The model under review builds one solid part; all positions refer to its coordinate system, in mm. Face numbers are marked on the shaded views. A direction names the side the tool comes from. Coordinates: 2 decimals unless noted, no trailing zeros. Loops run counter-clockwise (first coordinate to the right, second up) from the corner with the lowest first, then second, coordinate; pieces in that order, holes last. Notation, with made-up numbers: M 83.5,9 L 107.5,9 A26 cw 107.5,47 Z; hole C 80,20.5 d6. An arc over 180 degrees is marked long. Return JSON: item names as keys, results as strings.
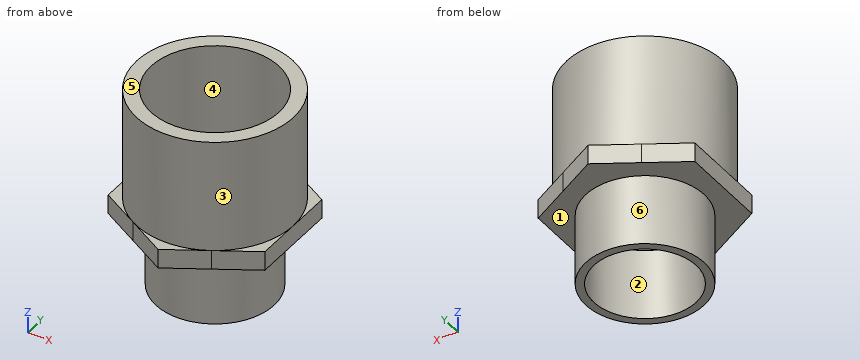
```python
from build123d import *

# Parameters (mm, degrees)
F3_DEPTH = 6


with BuildPart() as f1:
    # F0 (on Front) → F1 (revolve)
    with BuildSketch(Plane.XZ):
        Polygon((-18.5, 0), (-16, 0), (-16, 22), (-20, 28), (-20, 63), (-24.5, 63), (-24.5, 28), (-24.5, 22), (-18.5, 22), align=None)
    revolve(axis=Axis((0, 0, 64.797089), (0, 0, 1)))

    # F2 (on face) → F3 (join)
    with BuildSketch(Plane(origin=(0, 0, 22), x_dir=(1, 0, 0), z_dir=(0, 0, -1))):
        with BuildLine():
            Line((24.5, -14.145082), (24.5, 0))
            ThreePointArc((24.5, 0), (21.217622, -12.25), (12.25, -21.217622))
            Line((12.25, -21.217622), (24.5, -14.145082))
        make_face()
        with BuildLine():
            ThreePointArc((12.25, 21.217622), (21.217622, 12.25), (24.5, 0))
            Line((24.5, 0), (24.5, 14.145082))
            Line((24.5, 14.145082), (12.25, 21.217622))
        make_face()
        with BuildLine():
            ThreePointArc((-12.249999, 21.217623), (0, 24.5), (12.25, 21.217622))
            Line((12.25, 21.217622), (0, 28.290163))
            Line((0, 28.290163), (-12.249999, 21.217623))
        make_face()
        with BuildLine():
            Line((0, -28.290163), (12.25, -21.217622))
            ThreePointArc((12.25, -21.217622), (0, -24.5), (-12.25, -21.217622))
            Line((-12.25, -21.217622), (0, -28.290163))
        make_face()
        with BuildLine():
            ThreePointArc((-24.5, 0), (-21.217622, 12.25), (-12.249999, 21.217623))
            Line((-12.249999, 21.217623), (-24.5, 14.145082))
            Line((-24.5, 14.145082), (-24.5, 0))
        make_face()
        with BuildLine():
            Line((-24.5, -14.145082), (-12.25, -21.217622))
            ThreePointArc((-12.25, -21.217622), (-21.217622, -12.25), (-24.5, 0))
            Line((-24.5, 0), (-24.5, -14.145082))
        make_face()
    extrude(amount=-F3_DEPTH)

    # F4 (on Front) → F5 (revolve, cut)
    with BuildSketch(Plane.XZ):
        Polygon((-20, 28), (-16, 22), (0, 22), (0, 28), (-12.25, 28), align=None)
    revolve(axis=Axis((0, 0, 34.552477), (0, 0, 1)), mode=Mode.SUBTRACT)


solid = f1.part
```
1. Add section B-B on y = -23.5. Give the boundary of the cut face in (x, z).
Check values:
{"outline": "M -8.3,22 L 8.3,22 L 8.3,28 L 6.93,28 L 6.93,63 L -6.93,63 L -6.93,28 L -8.3,28 Z"}
2. The part is to be moulded in two halves that separate along X. For the marked faces 4, 5 and 6, say which applies: released by +X, released by -X, zero draft, split by the parting line, or undercut.
Check values:
{"face 4": "undercut", "face 5": "zero draft", "face 6": "split by the parting line"}
3. Add section D-D on z = 4. Give the boundary of the cut face in (x, y).
Check values:
{"outline": "C 0,0 d37; hole C 0,0 d32"}
4. Add section C-C on z = 51.5. Give the boundary of the cut face in (x, y).
Check values:
{"outline": "C 0,0 d49; hole C 0,0 d40"}
5. To check wall thickness, follow line 1 (X direction, y = 0, z = 45); line 2 (Y direction, x = 0, z = 14.5). State the ranges of each line that lie inside material, in increasing order.
Check values:
{"line 1": "-24.5 to -20, 20 to 24.5", "line 2": "-18.5 to -16, 16 to 18.5"}
6. Insertion check: pin 1 Ø1 at (x, z) = (2, 20) entering from -Y; pin 2 Ø8 at (x, z) = (8, 20) entering from +Y; pin 3 Ø4 at (x, z) = (-5.5, 40.5) entering from +Y. Each pin has a flat end and moves straight along its axis. Give the tip position at first contact, or say it passes through.
Check values:
{"pin 1": "y = -18.44", "pin 2": "y = 25.67", "pin 3": "y = 24.25"}
7. Machinability: for the marked faces 1, 2 and 3, which of the approach directions +Z, -Z, +X, -X, +Y, -Y give a long, thin tool a straight path to every point of the face, cutting with its end or side? Answer none if there is none.
Check values:
{"face 1": "-Z", "face 2": "+Z, -Z", "face 3": "+Z"}
8. Add section A-A on z = 25.5. Give the boundary of the cut face in (x, y).
Check values:
{"outline": "M -24.5,-14.15 L 0,-28.29 L 24.5,-14.15 L 24.5,14.15 L 0,28.29 L -24.5,14.15 Z; hole C 0,0 d36.67"}
